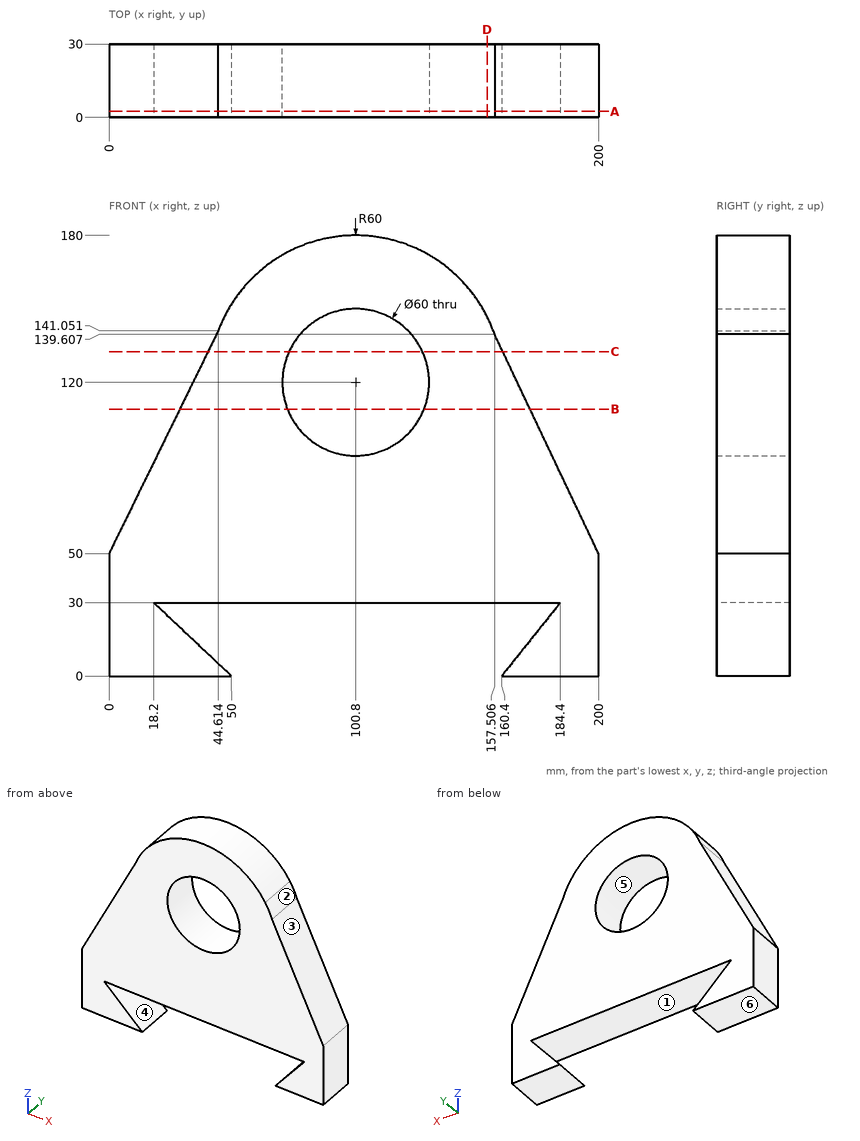
Input: dimensioned drawing with shaded views. Units: mm. Origin: part minimum x, y, z. A direction names the side the tool comes from. Round coordinates to 2 decimals unless told otherwise and drop trailing zeros. Order: outer loops, then holes, each group sorted by start corner. A loop starts at its lowest first (then second) coordinate and runs counter-clockwise, first axis right, second up. Notation, with made-up numbers: (82, 49.25) - (128, 49.25) arc R13 ccw to (128, 63.25) - close; hole circle Ø10 at (44.5, 25.5). An arc over 180 degrees is marked (long way). Use CSV: the item, a comma, the result in double quotes. Start each with the question number.
Q1. Section query C-C (z = 132.5). Return loops of the section in (x, y), and give its area (3 significant figures).
Q2. First-contact query: pin 1 (5 mm diameter, centred on y = 20.5, z = 75.5, fed in from -X); pin 2 (10 mm diameter, centred on y = 4.5, z = 70, fed in from +X); pin 3 (9 mm diameter, centred on x = 94.5, y = 11.5, fed in from -Z). Flat tips, straight axial feed; report the tip coordinate or a pass-through.
Q3. Material intervals for line 1 along Z through (x, y) = (99.5, 25.75) (1 decimal); line 2 along X through (y, z) = (19.5, 93) (1 decimal); line 3 along X through (y, z) = (15.75, 109), sorted ascending. Write a range as from..to.
Q4. Section query A-A (y = 2.5). Return loops of the section in (x, z) (1 decimal), and give its area (3 significant figures).
Q5. Access query for the marked faces 1 and 2. Directions: +Z, -Z, +X, -X, +Y, -Y. A direction counts if a zero-diameter tool reaches every point of the face in a straight line with its end or side. Return the directions, or none.
Q6. Section query B-B (z = 109). Return loops of the section in (x, y).
Q7. Section query D-D (x = 154.5). Return loops of the section in (y, z).
Q8. Mould query, pull axis Z, two halves, no side actions, for the marked faces 3, 4, 5 and 6. Classes: +Z half, -Z half, draft (parallel to the pull), parting line (faces both ways), or undercut.
Result set:
1,outline,"(40.42, 0) - (73.53, 0) - (73.53, 30) - (40.42, 30) - close; (128.07, 0) - (160.88, 0) - (160.88, 30) - (128.07, 30) - close"
1,area,"1,980 mm2"
2,pin 1,"stops at x = 11.27"
2,pin 2,"stops at x = 192.89"
2,pin 3,"stops at z = 30"
3,line 1,"z = 30..90, 150..180"
3,line 2,"x = 21.1..87.7, 113.9..179.6"
3,line 3,"x = 28.91..72.89, 128.71..172.02"
4,outline,"(0, 0) - (50, 0) - (18.2, 30) - (184.4, 30) - (160.4, 0) - (200, 0) - (200, 50) - (157.5, 139.6) arc R60 ccw to (151.9, 151.5) arc R60 ccw to (49.7, 151.5) arc R60 ccw to (44.6, 141.1) - (0, 50) - close; hole circle Ø60 at (100.8, 120)"
4,area,"20,400 mm2"
5,face 1,"+Y, -Y"
5,face 2,"+Z, +X, +Y, -Y"
6,outline,"(28.91, 0) - (72.89, 0) - (72.89, 30) - (28.91, 30) - close; (128.71, 0) - (172.02, 0) - (172.02, 30) - (128.71, 30) - close"
7,outline,"(0, 30) - (30, 30) - (30, 146.76) - (0, 146.76) - close"
8,face 3,"+Z half"
8,face 4,"undercut"
8,face 5,"undercut"
8,face 6,"-Z half"
